from build123d import *

# Parameters (mm, degrees)
F1_DEPTH = 5
F3_DEPTH = 1.5


with BuildPart() as f1:
    # F0 (on Top) → F1 (new body, symmetric)
    with BuildSketch(Plane.XY):
        with BuildLine():
            ThreePointArc((-5, 19.319071), (-5.707107, 19.026177), (-6, 18.319071))
            Line((-6, 18.319071), (-6, -35))
            ThreePointArc((-6, -35), (-4.242641, -39.242641), (0, -41))
            ThreePointArc((0, -41), (4.242641, -39.242641), (6, -35))
            Line((6, -35), (6, 35))
            ThreePointArc((6, 35), (4.242641, 39.242641), (0, 41))
            ThreePointArc((0, 41), (-4.242641, 39.242641), (-6, 35))
            Line((-6, 35), (-6, 30.319071))
            ThreePointArc((-6, 30.319071), (-5.707107, 29.611964), (-5, 29.319071))
            Line((-5, 29.319071), (1, 29.319071))
            ThreePointArc((1, 29.319071), (1.707107, 29.026177), (2, 28.319071))
            Line((2, 28.319071), (2, 20.319071))
            ThreePointArc((2, 20.319071), (1.707107, 19.611964), (1, 19.319071))
            Line((1, 19.319071), (-5, 19.319071))
        make_face()
    extrude(amount=F1_DEPTH, both=True)

    # F2 (on face) → F3 (cut, symmetric)
    with BuildSketch(Plane.XY.offset(5)):
        with BuildLine():
            Line((-4, 12.319071), (-4, -35))
            ThreePointArc((-4, -35), (-2.828427, -37.828427), (0, -39))
            ThreePointArc((0, -39), (3.145296, -37.471258), (3.886418, -34.053558))
            Line((3.886418, -34.053558), (3.886418, 12.319071))
            ThreePointArc((3.886418, 12.319071), (2.734853, 15.127347), (-0.056791, 16.318667))
            ThreePointArc((-0.056791, 16.318667), (-2.848435, 15.127347), (-4, 12.319071))
        make_face()
    extrude(amount=F3_DEPTH, both=True, mode=Mode.SUBTRACT)


solid = f1.part
Verification items for the finished model (mm, model axes). A direction names the side the tool comes from. Round coordinates to 2 decimals unless told otherwise and drop trailing zeros. Order: outer loops, then holes, each group sorted by start corner. A loop starts at its lowest first (then second) coordinate and runs counter-clockwise, first axis right, second up.
1. Access from +Z, -Z, +X, -X, +Y, -Y to the whole of each face (thin tool, end or side, straight path). Record for faces 1 (the flat face through (-2, 29.319, 0)), 2 (the flat face through (0, 1, -5)), 3 (the cylindrical face through (2.765, 15.096, 4.26)).
Final values:
face 1: +Z, -Z, -X
face 2: -Z, +X, -X, +Y, -Y
face 3: +Z
2. Section check A-A on z = 4.25. Record the cut outline in (x, y), then the cut area to 3 significant figures.
Final values:
outline: (-6, -35) arc R6 ccw to (0, -41) arc R6 ccw to (6, -35) - (6, 35) arc R6 ccw to (0, 41) arc R6 ccw to (-6, 35) - (-6, 30.32) arc R1 ccw to (-5, 29.32) - (1, 29.32) arc R1 cw to (2, 28.32) - (2, 20.32) arc R1 cw to (1, 19.32) - (-5, 19.32) arc R1 ccw to (-6, 18.32) - close; hole (-4, -35) arc R4 ccw to (0, -39) arc R4 ccw to (3.89, -34.05) - (3.89, 12.32) arc R4 ccw to (-0.06, 16.32) arc R4 ccw to (-4, 12.32) - close
area: 450 mm2
3. Go/stop test with flat-tipped pins: P1, Ø3, axis at x = -3, z = -2.5, coming from the +Y side; P2, Ø1.5, axis at x = -1, y = 13.5, coming from the +Z side; P3, Ø4, axis at y = 24.5, z = -0.5, coming from the -X side. Record where each tip stops, or that it passes through.
Final values:
P1: stops at y = 40.81
P2: stops at z = 3.5
P3: stops at x = 2
4. Section check D-D on x = -2. Record the cut outline in (y, z), then the cut area to 3 significant figures.
Final values:
outline: (-40.66, -5) - (19.32, -5) - (19.32, 5) - (15.78, 5) - (15.78, 3.5) - (-38.46, 3.5) - (-38.46, 5) - (-40.66, 5) - close; (29.32, -5) - (40.66, -5) - (40.66, 5) - (29.32, 5) - close
area: 632 mm2
5. Thickness scan on L1, parallel to Y at x = 1.5, z = 4.25; L2, parallel to Y at x = -0.25, z = 1.5; L3, parallel to Y at x = -2.25, z = 4.25. Record the ranges inside material, lowest first.
Final values:
L1: y = -40.81 to -38.71, 15.98 to 19.45, 29.19 to 40.81
L2: y = -40.99 to 19.32, 29.32 to 40.99
L3: y = -40.56 to -38.31, 15.63 to 19.32, 29.32 to 40.56
6. Release check for a two-part mould opening along Y. For faces 4 (the flat face through (-4, -11, 4)), 5 (the flat face through (-6, 33, 0)) record: +Y half, -Y half, draft (parallel to the pull), parting line (faces both ways), or undercut.
Final values:
face 4: undercut
face 5: draft
7. Section check B-B on y = -29.5. Record the cut outline in (x, z), then the cut area to 3 significant figures.
Final values:
outline: (-6, -5) - (6, -5) - (6, 5) - (3.89, 5) - (3.89, 3.5) - (-4, 3.5) - (-4, 5) - (-6, 5) - close
area: 108 mm2
8. Section check C-C on z = -4. Record the cut outline in (x, y), then the cut area to 3 significant figures.
Final values:
outline: (-6, -35) arc R6 ccw to (0, -41) arc R6 ccw to (6, -35) - (6, 35) arc R6 ccw to (0, 41) arc R6 ccw to (-6, 35) - (-6, 30.32) arc R1 ccw to (-5, 29.32) - (1, 29.32) arc R1 cw to (2, 28.32) - (2, 20.32) arc R1 cw to (1, 19.32) - (-5, 19.32) arc R1 ccw to (-6, 18.32) - close
area: 873 mm2
